Can you work these out from the model? Positions are in its coordinate system, mm. A direction names the side the tool comes from. Give positions to 0.01 mm unless a question says otherwise; leave off trailing zeros. Order: outer loops, then holes, each group sorted by start corner. A loop starts at its lowest first (then second) coordinate and runs counter-clockwise, first axis right, second up. Notation, with made-up numbers: (64, 29) - (90, 29) arc R26 ccw to (90, 55) - close; hole circle Ø2 at (87.25, 1.5). An arc over 180 degrees is marked (long way). One line per question, with ' | ' between items.
```python
from build123d import *

# Parameters (mm, degrees)
SKETCH1_R           = 17.5
SKETCH1_R_2         = 5
SKETCH1_R_3         = 2
BOSS_EXTRUDE1_DEPTH = 50
SKETCH2_R           = 20.5
SKETCH2_R_2         = 5
SKETCH2_R_3         = 2
BOSS_EXTRUDE2_DEPTH = 5
SKETCH3_R           = 20.5
SKETCH3_R_2         = 5
SKETCH3_R_3         = 2
BOSS_EXTRUDE3_DEPTH = 5


with BuildPart() as part:
    # Sketch1 → Boss-Extrude1 (new body)
    with BuildSketch(Plane.XY):
        Circle(SKETCH1_R)
        Circle(SKETCH1_R_2, mode=Mode.SUBTRACT)
        with Locations((0, 10)):
            Circle(SKETCH1_R_3, mode=Mode.SUBTRACT)
        with Locations((10, 0)):
            Circle(SKETCH1_R_3, mode=Mode.SUBTRACT)
        with Locations((0, -10)):
            Circle(SKETCH1_R_3, mode=Mode.SUBTRACT)
        with Locations((-10, 0)):
            Circle(SKETCH1_R_3, mode=Mode.SUBTRACT)
    extrude(amount=BOSS_EXTRUDE1_DEPTH)

    # Sketch2 → Boss-Extrude2 (add)
    with BuildSketch(Plane.XY.offset(50)):
        Circle(SKETCH2_R)
        Circle(SKETCH2_R_2, mode=Mode.SUBTRACT)
        with Locations((0, 10)):
            Circle(SKETCH2_R_3, mode=Mode.SUBTRACT)
        with Locations((10, 0)):
            Circle(SKETCH2_R_3, mode=Mode.SUBTRACT)
        with Locations((0, -10)):
            Circle(SKETCH2_R_3, mode=Mode.SUBTRACT)
        with Locations((-10, 0)):
            Circle(SKETCH2_R_3, mode=Mode.SUBTRACT)
    extrude(amount=BOSS_EXTRUDE2_DEPTH)

    # Sketch3 → Boss-Extrude3 (add)
    with BuildSketch(Plane(origin=(0, 0, 0), x_dir=(-1, 0, 0), z_dir=(0, 0, -1))):
        Circle(SKETCH3_R)
        Circle(SKETCH3_R_2, mode=Mode.SUBTRACT)
        with Locations((0, 10)):
            Circle(SKETCH3_R_3, mode=Mode.SUBTRACT)
        with Locations((10, 0)):
            Circle(SKETCH3_R_3, mode=Mode.SUBTRACT)
        with Locations((0, -10)):
            Circle(SKETCH3_R_3, mode=Mode.SUBTRACT)
        with Locations((-10, 0)):
            Circle(SKETCH3_R_3, mode=Mode.SUBTRACT)
    extrude(amount=BOSS_EXTRUDE3_DEPTH)


solid = part.part
```
(1) On a 3-axis mill with a long thin cutter (end or side, diameter ignored), from which of +Z, -Z, +X, -X, +Y, -Y can I reach the whole of each face in a straight line? I mean faces 4 (the face through (4, -4, 55)), 5 (the face through (-13.887, -10.648, 24.65)). Say none if no direction works.
Answer below:
face 4: +Z, +X, -X, +Y, -Y | face 5: none
(2) Imagine slicing it at A-A (x = 0). List the corners of the cut face in (y, z) for me.
Answer below:
outline: (-20.5, -5) - (-12, -5) - (-12, 55) - (-20.5, 55) - (-20.5, 50) - (-17.5, 50) - (-17.5, 0) - (-20.5, 0) - close; (-8, -5) - (-5, -5) - (-5, 55) - (-8, 55) - close; (5, -5) - (8, -5) - (8, 55) - (5, 55) - close; (12, -5) - (20.5, -5) - (20.5, 0) - (17.5, 0) - (17.5, 50) - (20.5, 50) - (20.5, 55) - (12, 55) - close
(3) Imagine slicing it at D-D (y = 11). List the corners of the cut face in (x, z) for me.
Answer below:
outline: (-17.3, -5) - (-1.73, -5) - (-1.73, 55) - (-17.3, 55) - (-17.3, 50) - (-13.61, 50) - (-13.61, 0) - (-17.3, 0) - close; (1.73, -5) - (17.3, -5) - (17.3, 0) - (13.61, 0) - (13.61, 50) - (17.3, 50) - (17.3, 55) - (1.73, 55) - close
(4) Imagine slicing it at C-C (z = 44.5). List the corners of the cut face in (x, y) for me.
Answer below:
outline: circle Ø35 at (0, 0); hole circle Ø4 at (-10, 0); hole circle Ø10 at (0, 0); hole circle Ø4 at (0, -10); hole circle Ø4 at (0, 10); hole circle Ø4 at (10, 0)
(5) If I drill on line 1 (Y direction, x = 0, z = 12); line 2 (Y direction, x = 0, z = -2); line 3 (Z direction, x = 17, y = 10), over which ranges is the centre line in solid material (lowest first)?
Answer below:
line 1: -17.5 to -12, -8 to -5, 5 to 8, 12 to 17.5 | line 2: -20.5 to -12, -8 to -5, 5 to 8, 12 to 20.5 | line 3: -5 to 0, 50 to 55
(6) Will these pins go through, and if not, where does the flat tip stop? pin 1 (6.5 mm diameter, centred on x = 0, y = -10, fed in from +Z); pin 2 (3 mm diameter, centred on x = 0, y = -10, fed in from -Z); pin 3 (6 mm diameter, centred on x = 11, z = 38, fed in from +Y); pin 4 (1.5 mm diameter, centred on x = -8, z = 8, fed in from -Y).
Answer below:
pin 1: z = 55 | pin 2: through | pin 3: y = 15.56 | pin 4: y = -15.93
(7) If we mould it in two halves opening along Z, with no side actions, what happens to faces 1 (the face through (15.1, 9.2, 50)), 2 (the face through (-4, -4, -5)), 3 (the face through (-4.444, -20.013, 52.465))? For each: released by +Z, released by -Z, zero draft, split by the parting line, or undercut.
Answer below:
face 1: undercut | face 2: released by -Z | face 3: zero draft
